Autodesk Inventor part; units mm, degrees
ref_plane "YZ Plane" through (0, 0, 0) normal (1, 0, 0) x (0, 1, 0)
ref_plane "XZ Plane" through (0, 0, 0) normal (0, 1, 0) x (-1, 0, 0)
ref_plane "XY Plane" through (0, 0, 0) normal (0, 0, 1) x (1, 0, 0)
sketch "Sketch1" plane through (0, 0, 0) normal (1, 0, 0) x (0, 1, 0)
  circle A0 centre (0, 0) radius 63.5
  arc A1 (51.7144, -18.8225) -> (30.3724, 0) centre (30.3724, -21.5106) ccw construction
  arc A2 (52.8957, -18.6737) -> (30.3724, 1.1906) centre (30.3724, -21.5106) ccw
  arc A3 (50.5331, -18.9713) -> (30.3724, -1.1906) centre (30.3724, -21.5106) ccw
  arc A4 (50.5331, -18.9713) -> (52.8957, -18.6737) centre (51.7144, -18.8225) ccw
  arc A5 (30.3724, 1.1906) -> (30.3724, -1.1906) centre (30.3724, 0) ccw
  line L0 (51.7144, -18.8225) -> (59.6705, -21.7183) construction
  line L1 (30.3724, 0) -> (63.5, 0) construction
  arc A6 (54.981, 2.4005) -> (28.0605, 11.623) centre (36.2922, -8.2502) ccw construction
  arc A7 (56.0154, 2.99) -> (27.6048, 12.723) centre (36.2922, -8.2502) ccw
  arc A8 (53.9465, 1.811) -> (28.5161, 10.523) centre (36.2922, -8.2502) ccw
  arc A9 (53.9465, 1.811) -> (56.0154, 2.99) centre (54.981, 2.4005) ccw
  arc A10 (27.6048, 12.723) -> (28.5161, 10.523) centre (28.0605, 11.623) ccw
  line L2 (54.981, 2.4005) -> (63.4396, 2.7698) construction
  line L3 (28.0605, 11.623) -> (58.6664, 24.3004) construction
  arc A11 (49.8771, 23.2581) -> (21.4765, 21.4765) centre (36.6869, 6.2662) ccw construction
  arc A12 (50.6072, 24.1986) -> (20.6346, 22.3184) centre (36.6869, 6.2662) ccw
  arc A13 (49.147, 22.3176) -> (22.3184, 20.6346) centre (36.6869, 6.2662) ccw
  arc A14 (49.147, 22.3176) -> (50.6072, 24.1986) centre (49.8771, 23.2581) ccw
  arc A15 (20.6346, 22.3184) -> (22.3184, 20.6346) centre (21.4765, 21.4765) ccw
  line L4 (49.8771, 23.2581) -> (57.5505, 26.8363) construction
  line L5 (21.4765, 21.4765) -> (44.9013, 44.9013) construction
  arc A16 (37.18, 40.5748) -> (11.623, 28.0605) centre (31.4962, 19.8287) ccw construction
  arc A17 (37.4946, 41.7231) -> (10.523, 28.5161) centre (31.4962, 19.8287) ccw
  arc A18 (36.8654, 39.4265) -> (12.723, 27.6048) centre (31.4962, 19.8287) ccw
  arc A19 (36.8654, 39.4265) -> (37.4946, 41.7231) centre (37.18, 40.5748) ccw
  arc A20 (10.523, 28.5161) -> (12.723, 27.6048) centre (11.623, 28.0605) ccw
  line L6 (37.18, 40.5748) -> (42.9, 46.8171) construction
  line L7 (11.623, 28.0605) -> (24.3004, 58.6664) construction
  arc A21 (18.8225, 51.7144) -> (0, 30.3724) centre (21.5106, 30.3724) ccw construction
  arc A22 (18.6737, 52.8957) -> (-1.1906, 30.3724) centre (21.5106, 30.3724) ccw
  arc A23 (18.9713, 50.5331) -> (1.1906, 30.3724) centre (21.5106, 30.3724) ccw
  arc A24 (18.9713, 50.5331) -> (18.6737, 52.8957) centre (18.8225, 51.7144) ccw
  arc A25 (-1.1906, 30.3724) -> (1.1906, 30.3724) centre (0, 30.3724) ccw
  line L8 (18.8225, 51.7144) -> (21.7183, 59.6705) construction
  line L9 (0, 30.3724) -> (0, 63.5) construction
  arc A26 (-2.4005, 54.981) -> (-11.623, 28.0605) centre (8.2502, 36.2922) ccw construction
  arc A27 (-2.99, 56.0154) -> (-12.723, 27.6048) centre (8.2502, 36.2922) ccw
  arc A28 (-1.811, 53.9465) -> (-10.523, 28.5161) centre (8.2502, 36.2922) ccw
  arc A29 (-1.811, 53.9465) -> (-2.99, 56.0154) centre (-2.4005, 54.981) ccw
  arc A30 (-12.723, 27.6048) -> (-10.523, 28.5161) centre (-11.623, 28.0605) ccw
  line L10 (-2.4005, 54.981) -> (-2.7698, 63.4396) construction
  line L11 (-11.623, 28.0605) -> (-24.3004, 58.6664) construction
  arc A31 (-23.2581, 49.8771) -> (-21.4765, 21.4765) centre (-6.2662, 36.6869) ccw construction
  arc A32 (-24.1986, 50.6072) -> (-22.3184, 20.6346) centre (-6.2662, 36.6869) ccw
  arc A33 (-22.3176, 49.147) -> (-20.6346, 22.3184) centre (-6.2662, 36.6869) ccw
  arc A34 (-22.3176, 49.147) -> (-24.1986, 50.6072) centre (-23.2581, 49.8771) ccw
  arc A35 (-22.3184, 20.6346) -> (-20.6346, 22.3184) centre (-21.4765, 21.4765) ccw
  line L12 (-23.2581, 49.8771) -> (-26.8363, 57.5505) construction
  line L13 (-21.4765, 21.4765) -> (-44.9013, 44.9013) construction
  arc A36 (-40.5748, 37.18) -> (-28.0605, 11.623) centre (-19.8287, 31.4962) ccw construction
  arc A37 (-41.7231, 37.4946) -> (-28.5161, 10.523) centre (-19.8287, 31.4962) ccw
  arc A38 (-39.4265, 36.8654) -> (-27.6048, 12.723) centre (-19.8287, 31.4962) ccw
  arc A39 (-39.4265, 36.8654) -> (-41.7231, 37.4946) centre (-40.5748, 37.18) ccw
  arc A40 (-28.5161, 10.523) -> (-27.6048, 12.723) centre (-28.0605, 11.623) ccw
  line L14 (-40.5748, 37.18) -> (-46.8171, 42.9) construction
  line L15 (-28.0605, 11.623) -> (-58.6664, 24.3004) construction
  arc A41 (-51.7144, 18.8225) -> (-30.3724, 0) centre (-30.3724, 21.5106) ccw construction
  arc A42 (-52.8957, 18.6737) -> (-30.3724, -1.1906) centre (-30.3724, 21.5106) ccw
  arc A43 (-50.5331, 18.9713) -> (-30.3724, 1.1906) centre (-30.3724, 21.5106) ccw
  arc A44 (-50.5331, 18.9713) -> (-52.8957, 18.6737) centre (-51.7144, 18.8225) ccw
  arc A45 (-30.3724, -1.1906) -> (-30.3724, 1.1906) centre (-30.3724, 0) ccw
  line L16 (-51.7144, 18.8225) -> (-59.6705, 21.7183) construction
  line L17 (-30.3724, 0) -> (-63.5, 0) construction
  arc A46 (-54.981, -2.4005) -> (-28.0605, -11.623) centre (-36.2922, 8.2502) ccw construction
  arc A47 (-56.0154, -2.99) -> (-27.6048, -12.723) centre (-36.2922, 8.2502) ccw
  arc A48 (-53.9465, -1.811) -> (-28.5161, -10.523) centre (-36.2922, 8.2502) ccw
  arc A49 (-53.9465, -1.811) -> (-56.0154, -2.99) centre (-54.981, -2.4005) ccw
  arc A50 (-27.6048, -12.723) -> (-28.5161, -10.523) centre (-28.0605, -11.623) ccw
  line L18 (-54.981, -2.4005) -> (-63.4396, -2.7698) construction
  line L19 (-28.0605, -11.623) -> (-58.6664, -24.3004) construction
  arc A51 (-49.8771, -23.2581) -> (-21.4765, -21.4765) centre (-36.6869, -6.2662) ccw construction
  arc A52 (-50.6072, -24.1986) -> (-20.6346, -22.3184) centre (-36.6869, -6.2662) ccw
  arc A53 (-49.147, -22.3176) -> (-22.3184, -20.6346) centre (-36.6869, -6.2662) ccw
  arc A54 (-49.147, -22.3176) -> (-50.6072, -24.1986) centre (-49.8771, -23.2581) ccw
  arc A55 (-20.6346, -22.3184) -> (-22.3184, -20.6346) centre (-21.4765, -21.4765) ccw
  line L20 (-49.8771, -23.2581) -> (-57.5505, -26.8363) construction
  line L21 (-21.4765, -21.4765) -> (-44.9013, -44.9013) construction
  arc A56 (-37.18, -40.5748) -> (-11.623, -28.0605) centre (-31.4962, -19.8287) ccw construction
  arc A57 (-37.4946, -41.7231) -> (-10.523, -28.5161) centre (-31.4962, -19.8287) ccw
  arc A58 (-36.8654, -39.4265) -> (-12.723, -27.6048) centre (-31.4962, -19.8287) ccw
  arc A59 (-36.8654, -39.4265) -> (-37.4946, -41.7231) centre (-37.18, -40.5748) ccw
  arc A60 (-10.523, -28.5161) -> (-12.723, -27.6048) centre (-11.623, -28.0605) ccw
  line L22 (-37.18, -40.5748) -> (-42.9, -46.8171) construction
  line L23 (-11.623, -28.0605) -> (-24.3004, -58.6664) construction
  arc A61 (-18.8225, -51.7144) -> (0, -30.3724) centre (-21.5106, -30.3724) ccw construction
  arc A62 (-18.6737, -52.8957) -> (1.1906, -30.3724) centre (-21.5106, -30.3724) ccw
  arc A63 (-18.9713, -50.5331) -> (-1.1906, -30.3724) centre (-21.5106, -30.3724) ccw
  arc A64 (-18.9713, -50.5331) -> (-18.6737, -52.8957) centre (-18.8225, -51.7144) ccw
  arc A65 (1.1906, -30.3724) -> (-1.1906, -30.3724) centre (0, -30.3724) ccw
  line L24 (-18.8225, -51.7144) -> (-21.7183, -59.6705) construction
  line L25 (0, -30.3724) -> (0, -63.5) construction
  arc A66 (2.4005, -54.981) -> (11.623, -28.0605) centre (-8.2502, -36.2922) ccw construction
  arc A67 (2.99, -56.0154) -> (12.723, -27.6048) centre (-8.2502, -36.2922) ccw
  arc A68 (1.811, -53.9465) -> (10.523, -28.5161) centre (-8.2502, -36.2922) ccw
  arc A69 (1.811, -53.9465) -> (2.99, -56.0154) centre (2.4005, -54.981) ccw
  arc A70 (12.723, -27.6048) -> (10.523, -28.5161) centre (11.623, -28.0605) ccw
  line L26 (2.4005, -54.981) -> (2.7698, -63.4396) construction
  line L27 (11.623, -28.0605) -> (24.3004, -58.6664) construction
  arc A71 (23.2581, -49.8771) -> (21.4765, -21.4765) centre (6.2662, -36.6869) ccw construction
  arc A72 (24.1986, -50.6072) -> (22.3184, -20.6346) centre (6.2662, -36.6869) ccw
  arc A73 (22.3176, -49.147) -> (20.6346, -22.3184) centre (6.2662, -36.6869) ccw
  arc A74 (22.3176, -49.147) -> (24.1986, -50.6072) centre (23.2581, -49.8771) ccw
  arc A75 (22.3184, -20.6346) -> (20.6346, -22.3184) centre (21.4765, -21.4765) ccw
  line L28 (23.2581, -49.8771) -> (26.8363, -57.5505) construction
  line L29 (21.4765, -21.4765) -> (44.9013, -44.9013) construction
  arc A76 (40.5748, -37.18) -> (28.0605, -11.623) centre (19.8287, -31.4962) ccw construction
  arc A77 (41.7231, -37.4946) -> (28.5161, -10.523) centre (19.8287, -31.4962) ccw
  arc A78 (39.4265, -36.8654) -> (27.6048, -12.723) centre (19.8287, -31.4962) ccw
  arc A79 (39.4265, -36.8654) -> (41.7231, -37.4946) centre (40.5748, -37.18) ccw
  arc A80 (28.5161, -10.523) -> (27.6048, -12.723) centre (28.0605, -11.623) ccw
  line L30 (40.5748, -37.18) -> (46.8171, -42.9) construction
  line L31 (28.0605, -11.623) -> (58.6664, -24.3004) construction
  dimension "d0" = 127
  dimension "d1" = 20
  dimension "d2" = 8.4667
  dimension "d5" = 2.3813
  dimension "d8" = 360
  dimension "d10" = 20.32
extrude "Plate1" add sketch "Sketch1" along normal blind 3.048
equation "\"d11\" = Thickness"
equation "\"BendRadius\" = Thickness"
equation "\"BendReliefWidth\" = Thickness"
equation "\"BendReliefDepth\" = 0.5 * Thickness"
equation "\"CornerReliefSize\" = 4 * Thickness"
equation "\"MinimumRemnant\" = 2 * Thickness"
equation "\"TransitionRadius\" = BendRadius"
equation "\"JacobiRadiusSize\" = BendRadius"
equation "\"GapSize\" = Thickness"
properties part number "FanCentRotorRear"
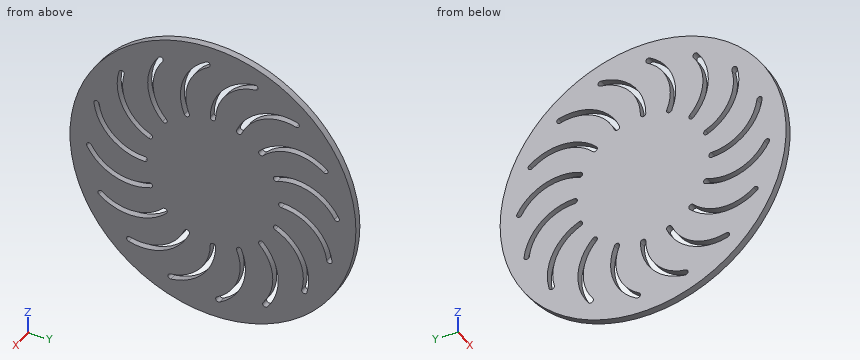
Could you check a few things on this model? Use its own coordinates, in mm. Give positions to 0.01 mm unless a question says otherwise; leave off trailing zeros. Write each loop counter-clockwise with the first axis right and the second up, starting at its lowest first coordinate (ties: lowest second). Pieces come first, ordered by that corner, then holes. Notation, with made-up numbers: (-33.5, -31) -> (-5.5, -31) arc R16 ccw to (-5.5, -24) -> close; hole circle Ø1 at (36, -22.5). An arc over 180 degrees is marked (long way). Answer as a JSON object with one key per item and string values.
Q1. Please list where these lines run through material, in increasing order: L1, parallel to Y at x = 2.5, z = -7; L2, parallel to Y at x = 1.75, z = -9; L3, parallel to Y at x = 1.5, z = 21.
Taken from the geometry:
{"L1": "y = -63.11 to -53.11, -49.72 to 44.6, 47.83 to 63.11", "L2": "y = -62.86 to -51.05, -47.03 to 46.38, 49.32 to 62.86", "L3": "y = -59.93 to -39.96, -37.23 to -22.68, -20.39 to 20.39, 22.69 to 59.93"}
Q2. Suppose I cut it at C-C on z = 16. Write out the boundary of the cut face in (x, y).
Taken from the geometry:
{"outline": "(0, -61.45) -> (3.05, -61.45) -> (3.05, -52.39) -> (0, -52.39) -> close; (0, -49.93) -> (3.05, -49.93) -> (3.05, -36.42) -> (0, -36.42) -> close; (0, -32.97) -> (3.05, -32.97) -> (3.05, 61.45) -> (0, 61.45) -> close"}
Q3. Suppose I cut it at B-B on z = 34.5. Write out the boundary of the cut face in (x, y), then the cut area to 3 significant figures.
Taken from the geometry:
{"outline": "(0, -53.31) -> (3.05, -53.31) -> (3.05, -42.33) -> (0, -42.33) -> close; (0, -39.93) -> (3.05, -39.93) -> (3.05, -28.86) -> (0, -28.86) -> close; (0, -26.47) -> (3.05, -26.47) -> (3.05, -14.38) -> (0, -14.38) -> close; (0, -11.99) -> (3.05, -11.99) -> (3.05, -0.81) -> (0, -0.81) -> close; (0, 1.61) -> (3.05, 1.61) -> (3.05, 14.17) -> (0, 14.17) -> close; (0, 17.44) -> (3.05, 17.44) -> (3.05, 53.31) -> (0, 53.31) -> close", "area": "286 mm²"}
Q4. Will these pins go through, and if not, where does the flat tip stop? pin 1 Ø1.5 at (x, y) = (1, 5) entering from +Z; pin 2 Ø1 at (x, z) = (1.5, 37.5) entering from -Y.
Taken from the geometry:
{"pin 1": "stops at z = 63.36", "pin 2": "stops at y = -51.61"}
Q5. Suppose I cut it at D-D on x = 1.2. Count the separate pieces of the cut face and the enclosed holes in it, then the cut area to 3 significant figures.
Taken from the geometry:
{"separate pieces": "1", "enclosed holes": "16", "area": "11,400 mm²"}
Q6. Suppose I cut it at A-A on y = 5. Write out the boundary of the cut face in (x, z), then the cut area to 3 significant figures.
Taken from the geometry:
{"outline": "(0, -63.3) -> (3.05, -63.3) -> (3.05, -54.73) -> (0, -54.73) -> close; (0, -51.7) -> (3.05, -51.7) -> (3.05, 42.22) -> (0, 42.22) -> close; (0, 45.95) -> (3.05, 45.95) -> (3.05, 63.3) -> (0, 63.3) -> close", "area": "365 mm²"}
